Source: CAD feature listing. Evaluate the final solid. Frame: model axes, mm. A direction names the side the tool comes from. Coordinates: 2 decimals unless noted, no trailing zeros. Write each loop counter-clockwise with the first axis right and the second up, starting at its lowest first coordinate (ties: lowest second). Pieces come first, ordered by that corner, then holes. Notation, with made-up numbers: (84.5, 34) -> (142.5, 34) arc R22 cw to (142.5, 61) -> close; hole circle Ø9 at (80.25, 69). An arc over 180 degrees is marked (long way). Write item = value, one per line.
from build123d import *

# Parameters (mm, degrees)
F1_DEPTH = 8
F6_DEPTH = 3
F7_DEPTH = 3
F8_DEPTH = 3
F9_DEPTH = 3
F10_R    = 3


with BuildPart() as f1:
    # F0 (on Top) → F1 (new body)
    with BuildSketch(Plane.XY):
        with BuildLine():
            ThreePointArc((-11.075, 0), (-7.8312076016, 7.8312076016), (0, 11.075))
            Line((0, 11.075), (0, 15))
            ThreePointArc((0, 15), (-2.5365296809, 14.7839783948), (-5, 14.1421356237))
            ThreePointArc((-5, 14.1421356237), (-10.6066017178, 10.6066017178), (-14.1421356237, 5))
            ThreePointArc((-14.1421356237, 5), (-14.7839783948, 2.5365296809), (-15, 0))
            Line((-15, 0), (-11.075, 0))
        make_face()
        with BuildLine():
            Line((0, -15), (0, -11.075))
            ThreePointArc((0, -11.075), (-7.8312076016, -7.8312076016), (-11.075, 0))
            Line((-11.075, 0), (-15, 0))
            ThreePointArc((-15, 0), (-14.7839783948, -2.5365296809), (-14.1421356237, -5))
            ThreePointArc((-14.1421356237, -5), (-10.6066017178, -10.6066017178), (-5, -14.1421356237))
            ThreePointArc((-5, -14.1421356237), (-2.5365296809, -14.7839783948), (0, -15))
        make_face()
        with BuildLine():
            ThreePointArc((-14.1421356237, -5), (-14.7839783948, -2.5365296809), (-15, 0))
            Line((-15, 0), (-21, 0))
            Line((-21, 0), (-21, -5))
            Line((-21, -5), (-14.1421356237, -5))
        make_face()
        with BuildLine():
            Line((-21, 0), (-15, 0))
            ThreePointArc((-15, 0), (-14.7839783948, 2.5365296809), (-14.1421356237, 5))
            Line((-14.1421356237, 5), (-21, 5))
            Line((-21, 5), (-21, 0))
        make_face()
        with BuildLine():
            ThreePointArc((-5, 14.1421356237), (-2.5365296809, 14.7839783948), (0, 15))
            Line((0, 15), (0, 21))
            Line((0, 21), (-5, 21))
            Line((-5, 21), (-5, 14.1421356237))
        make_face()
        with BuildLine():
            ThreePointArc((0, 11.075), (7.8312076016, 7.8312076016), (11.075, 0))
            Line((11.075, 0), (15, 0))
            ThreePointArc((15, 0), (14.7839783948, 2.5365296809), (14.1421356237, 5))
            ThreePointArc((14.1421356237, 5), (10.6066017178, 10.6066017178), (5, 14.1421356237))
            ThreePointArc((5, 14.1421356237), (2.5365296809, 14.7839783948), (0, 15))
            Line((0, 15), (0, 11.075))
        make_face()
        with BuildLine():
            Line((15, 0), (11.075, 0))
            ThreePointArc((11.075, 0), (7.8312076016, -7.8312076016), (0, -11.075))
            Line((0, -11.075), (0, -15))
            ThreePointArc((0, -15), (2.5365296809, -14.7839783948), (5, -14.1421356237))
            ThreePointArc((5, -14.1421356237), (10.6066017178, -10.6066017178), (14.1421356237, -5))
            ThreePointArc((14.1421356237, -5), (14.7839783948, -2.5365296809), (15, 0))
        make_face()
        with BuildLine():
            ThreePointArc((5, -14.1421356237), (2.5365296809, -14.7839783948), (0, -15))
            Line((0, -15), (0, -21))
            Line((0, -21), (5, -21))
            Line((5, -21), (5, -14.1421356237))
        make_face()
        with BuildLine():
            Line((0, -21), (0, -15))
            ThreePointArc((0, -15), (-2.5365296809, -14.7839783948), (-5, -14.1421356237))
            Line((-5, -14.1421356237), (-5, -21))
            Line((-5, -21), (0, -21))
        make_face()
        with BuildLine():
            Line((21, 0), (15, 0))
            ThreePointArc((15, 0), (14.7839783948, -2.5365296809), (14.1421356237, -5))
            Line((14.1421356237, -5), (21, -5))
            Line((21, -5), (21, 0))
        make_face()
        with BuildLine():
            ThreePointArc((14.1421356237, 5), (14.7839783948, 2.5365296809), (15, 0))
            Line((15, 0), (21, 0))
            Line((21, 0), (21, 5))
            Line((21, 5), (14.1421356237, 5))
        make_face()
        with BuildLine():
            Line((0, 21), (0, 15))
            ThreePointArc((0, 15), (2.5365296809, 14.7839783948), (5, 14.1421356237))
            Line((5, 14.1421356237), (5, 21))
            Line((5, 21), (0, 21))
        make_face()
    extrude(amount=F1_DEPTH)

    # F5 (on face) → F6 (cut)
    with BuildSketch(Plane.XZ.offset(21)):
        with BuildLine():
            Line((0, 7.55), (0, 0.45))
            ThreePointArc((0, 0.45), (2.5102290732, 1.4897709268), (3.55, 4))
            ThreePointArc((3.55, 4), (2.5102290732, 6.5102290732), (0, 7.55))
        make_face()
        with BuildLine():
            ThreePointArc((0, 7.55), (-3.55, 4), (0, 0.45))
            Line((0, 0.45), (0, 7.55))
        make_face()
    extrude(amount=-F6_DEPTH, mode=Mode.SUBTRACT)

    # F2 (on face) → F7 (cut)
    with BuildSketch(Plane(origin=(-21, 0, 0), x_dir=(0, -1, 0), z_dir=(-1, 0, 0))):
        with BuildLine():
            ThreePointArc((0, 7.55), (-3.55, 4), (0, 0.45))
            Line((0, 0.45), (0, 7.55))
        make_face()
        with BuildLine():
            Line((0, 7.55), (0, 0.45))
            ThreePointArc((0, 0.45), (2.5102290732, 1.4897709268), (3.55, 4))
            ThreePointArc((3.55, 4), (2.5102290732, 6.5102290732), (0, 7.55))
        make_face()
    extrude(amount=-F7_DEPTH, mode=Mode.SUBTRACT)

    # F3 (on face) → F8 (cut)
    with BuildSketch(Plane(origin=(0, 21, 0), x_dir=(-1, 0, 0), z_dir=(0, 1, 0))):
        with BuildLine():
            ThreePointArc((0, 7.55), (-3.55, 4), (0, 0.45))
            Line((0, 0.45), (0, 7.55))
        make_face()
        with BuildLine():
            Line((0, 7.55), (0, 0.45))
            ThreePointArc((0, 0.45), (2.5102290732, 1.4897709268), (3.55, 4))
            ThreePointArc((3.55, 4), (2.5102290732, 6.5102290732), (0, 7.55))
        make_face()
    extrude(amount=-F8_DEPTH, mode=Mode.SUBTRACT)

    # F4 (on face) → F9 (cut)
    with BuildSketch(Plane.YZ.offset(21)):
        with BuildLine():
            ThreePointArc((0, 7.55), (-3.55, 4), (0, 0.45))
            Line((0, 0.45), (0, 7.55))
        make_face()
        with BuildLine():
            Line((0, 7.55), (0, 0.45))
            ThreePointArc((0, 0.45), (2.5102290732, 1.4897709268), (3.55, 4))
            ThreePointArc((3.55, 4), (2.5102290732, 6.5102290732), (0, 7.55))
        make_face()
    extrude(amount=-F9_DEPTH, mode=Mode.SUBTRACT)

    # F10
    f10_edges = [f1.edges().sort_by_distance(p)[0] for p in [
        (-5, -17.571068, 0),
        (-5, -17.571068, 8),
        (5, -17.571068, 8),
        (5, -17.571068, 0),
        (-17.571068, 5, 8),
        (-17.571068, 5, 0),
        (-17.571068, -5, 8),
        (-17.571068, -5, 0),
        (5, 17.571068, 8),
        (5, 17.571068, 0),
        (17.571068, 5, 8),
        (17.571068, 5, 0),
        (17.571068, -5, 8),
        (17.571068, -5, 0),
        (-5, 17.571068, 8),
        (-5, 17.571068, 0),
    ]]
    fillet(f10_edges, radius=F10_R)


solid = f1.part
1) Cut plane B-B, the plane y = 10. Output: boundary loops of the cut face in (x, z), and give its area (3 significant figures).
Answer block:
outline = (-11.18, 0) -> (-4.76, 0) -> (-4.76, 8) -> (-11.18, 8) -> close; (4.76, 0) -> (11.18, 0) -> (11.18, 8) -> (4.76, 8) -> close
area = 103 mm2
2) First-contact query: pin 1 Ø0.6 at (y, z) = (-18.5, 4.5) entering from +X; pin 2 Ø1.6 at (x, z) = (-16, 4.5) entering from +Y; pin 3 Ø3 at (x, y) = (-7.5, -1.5) entering from +Z; pin 4 Ø1.6 at (y, z) = (18, 3.5) entering from -X. Flat tips, straight axial feed; report the tip coordinate or a pass-through.
Answer block:
pin_1 = 5
pin_2 = 5
pin_3 = through
pin_4 = -5
3) Reachability of faces 4 (the flat face through (-18, 5, 4)), 5 (the cylindrical face through (-4.1, 17.52, 7.14)), 6 (the cylindrical face through (-4.1, -17.62, 0.86)), 7 (the cylindrical face through (17.62, -4.1, 0.86)), 8 (the cylindrical face through (-4.1, 17.52, 0.86)) from +Z, -Z, +X, -X, +Y, -Y: full face, straight path, thin tool, end or side. Return the list, or none.
Answer block:
face_4 = +Z, -Z, -X, +Y
face_5 = +Z, -X, +Y
face_6 = -Z, -X, -Y
face_7 = -Z, +X, -Y
face_8 = -Z, -X, +Y
4) Material intervals for probe 1 along X at (y, z) = (-19, 4); probe 2 along Y at (x, z) = (14.5, 4.75); probe 3 along Y at (x, z) = (-9, 2.5), sorted ascending. Write a range as [from, to].
Answer block:
probe_1 = [-5, -3.55], [3.55, 5]
probe_2 = [-5, 5]
probe_3 = [-12, -6.45], [6.45, 12]
5) Pull-direction query (Y, two-part tool) for faces 1 (the cylindrical face through (-17.52, -4.1, 0.86)), 2 (the flat face through (18, 0, 4)), 3 (the cylindrical face through (17.52, 4.1, 0.86)); classes: +Y half, -Y half, draft (parallel to the pull), parting line (faces both ways), or undercut.
Answer block:
face_1 = -Y half
face_2 = undercut
face_3 = +Y half
6) Cut plane A-A, the plane x = 1. Output: boundary loops of the cut face in (y, z), and give its area (3 significant figures).
Answer block:
outline = (-21, 0) -> (-11.03, 0) -> (-11.03, 8) -> (-21, 8) -> (-21, 7.41) -> (-18, 7.41) -> (-18, 0.59) -> (-21, 0.59) -> close; (11.03, 0) -> (21, 0) -> (21, 0.59) -> (18, 0.59) -> (18, 7.41) -> (21, 7.41) -> (21, 8) -> (11.03, 8) -> close
area = 119 mm2
7) Cut plane C-C, the plane x = 9. Output: boundary loops of the cut face in (y, z), and give its area (3 significant figures).
Answer block:
outline = (-12, 0) -> (-6.45, 0) -> (-6.45, 8) -> (-12, 8) -> close; (6.45, 0) -> (12, 0) -> (12, 8) -> (6.45, 8) -> close
area = 88.7 mm2
